Here's how the part is built. I have some questions about the finished solid (model axes, mm). A direction names the side the tool comes from. Coordinates: 2 decimals unless noted, no trailing zeros. Order: outer loops, then holes, each group sorted by start corner. A loop starts at its lowest first (then second) coordinate and runs counter-clockwise, first axis right, second up. Notation, with made-up numbers: (18.25, 53) - (31.25, 53) arc R10 cw to (31.25, 58) - close; hole circle Ø7 at (-26.75, 45.5). An arc over 180 degrees is marked (long way). Answer as CSV lines item,"result". Start each with the question number.
Item 1: I'm going to push flat-ended pins straight in: pin 1 (8 mm diameter, centred on y = 0, z = 15, fed in from +X); pin 2 (5 mm diameter, centred on x = 15, z = 2, fed in from +Y); pin 3 (8 mm diameter, centred on y = -2, z = -6, fed in from +X). Where does each tip first touch, or does it pass through?
Item 2: Imagine slicing it at B-B on y = 42.8. List the corners of the cut face in (x, z) for me, and give its area (3 significant figures).
Item 3: Imagine slicing it at A-A on x = 24. List the corners of the cut face in (y, z) for me, and give its area (3 significant figures).
Item 4: I need wall thicknesses on line 1 (Z direction, x = 2, y = 0); line 2 (Y direction, x = 5, z = 15); line 3 (X direction, y = 1.5, z = 18). Which ranges of each line are inside material? Lowest first, please.
Item 5: Imagine slicing it at C-C on z = -6. List the corners of the cut face in (x, y) for me, and give its area (3 significant figures).
Item 6: We'd pull the mould along Z, two halves only. Please class faces 1 (the face through (24, 0, 32)), 2 (the face through (36, 0, -15)), 3 (the face through (24, 0, -28)): pulls with the +Z half, pulls with the -Z half, needs draft (parallel to the pull), parting line crosses it, or undercut.
Item 7: Imagine slicing it at D-D on x = 10. List the corners of the cut face in (y, z) for me, and give its area (3 significant figures).
Item 8: On a 3-axis mill with a long thin cutter (end or side, diameter ignored), from which of +Z, -Z, +X, -X, +Y, -Y can I reach the whole of each face in a straight line? I mean faces 4 (the face through (12, 0, 0)), 5 (the face through (46.998, 42, 0)), 6 (the face through (48.674, 25.571, 0.14)), 7 (the face through (-1.479, 0.165, 11.254)). Say none if no direction works.
from build123d import *

# Parameters (mm, degrees)
BOSS_EXTRUDE1_DEPTH      = 3.75
SKETCH2_R                = 3.75
BOSS_EXTRUDE2_DEPTH      = 3
M4_CLEARANCE_HOLE1_D     = 4.5
M4_CLEARANCE_HOLE1_DEPTH = 10
M4_CLEARANCE_HOLE1_TIP   = 1.351936393
CUT_EXTRUDE1_DEPTH       = 33
CUT_EXTRUDE1_DEPTH_BACK  = 33
BOSS_EXTRUDE3_DEPTH      = 10
M3_CLEARANCE_HOLE1_D     = 3.4
M3_CLEARANCE_HOLE1_DEPTH = 10
M3_CLEARANCE_HOLE1_TIP   = 1.021463052


with BuildPart() as part:
    # Sketch1 → Boss-Extrude1 (new body, symmetric)
    with BuildSketch(Plane(origin=(0, 0, 0), x_dir=(1, 0, 0), z_dir=(0, 1, 0))):
        with BuildLine():
            Line((0, -11), (12, -11))
            Line((12, -11), (12, 11))
            Line((12, 11), (0, 11))
            Line((0, 11), (0, 19))
            Line((0, 19), (12, 19))
            Line((12, 19), (12, 20))
            ThreePointArc((12, 20), (24, 32), (36, 20))
            Line((36, 20), (36, 10))
            Line((36, 10), (55, 10))
            Line((55, 10), (55, -10))
            Line((55, -10), (36, -10))
            Line((36, -10), (36, -20))
            ThreePointArc((36, -20), (24, -32), (12, -20))
            Line((12, -20), (12, -19))
            Line((12, -19), (0, -19))
            Line((0, -19), (0, -11))
        make_face()
        with BuildLine():
            Line((32, 20), (32, -20))
            ThreePointArc((32, -20), (24, -28), (16, -20))
            Line((16, -20), (16, 20))
            ThreePointArc((16, 20), (24, 28), (32, 20))
        make_face(mode=Mode.SUBTRACT)
    extrude(amount=BOSS_EXTRUDE1_DEPTH, both=True)

    # Sketch2 → Boss-Extrude2 (add)
    with BuildSketch(Plane.ZY):
        with Locations((-15, 0)):
            Circle(SKETCH2_R)
        with Locations((15, 0)):
            Circle(SKETCH2_R)
    extrude(amount=BOSS_EXTRUDE2_DEPTH)

    # M4 Clearance Hole1
    with Locations(Plane.ZY.offset(3)):
        with Locations((-15, 0), (15, 0)):
            Hole(M4_CLEARANCE_HOLE1_D / 2, depth=M4_CLEARANCE_HOLE1_DEPTH)
            with Locations((0, 0, -(M4_CLEARANCE_HOLE1_DEPTH + M4_CLEARANCE_HOLE1_TIP / 2))):  # 118° drill point
                Cone(0, M4_CLEARANCE_HOLE1_D / 2, M4_CLEARANCE_HOLE1_TIP, mode=Mode.SUBTRACT)

    # Sketch6 → Cut-Extrude1 (cut, two sides)
    with BuildSketch(Plane.XY) as cut_extrude1_sk:
        with BuildLine():
            Line((53.548387097, -7.31769585), (58.512723929, -6.476790348))
            Line((58.512723929, -6.476790348), (58.512723929, 16.833295116))
            Line((58.512723929, 16.833295116), (46.662820439, 16.833295116))
            ThreePointArc((46.662820439, 16.833295116), (46.996356715, 3.87133796), (53.548387097, -7.31769585))
        make_face()
    extrude(amount=CUT_EXTRUDE1_DEPTH, mode=Mode.SUBTRACT)
    extrude(cut_extrude1_sk.sketch, amount=-CUT_EXTRUDE1_DEPTH_BACK, mode=Mode.SUBTRACT)

    # Sketch7 → Boss-Extrude3 (add, symmetric)
    with BuildSketch(Plane.XY):
        with BuildLine():
            Line((46.662820439, 16.833295116), (50.743158051, 34.556424956))
            ThreePointArc((50.743158051, 34.556424956), (50.934151856, 35.670993937), (50.998088989, 36.8))
            Line((50.998088989, 36.8), (50.998088989, 53))
            Line((50.998088989, 53), (50.075012066, 52.615384615))
            ThreePointArc((50.075012066, 52.615384615), (47.837837517, 50.773500981), (46.998088989, 48))
            Line((46.998088989, 48), (46.998088989, 36.8))
            ThreePointArc((46.998088989, 36.8), (46.959726709, 36.122596362), (46.845130426, 35.453854973))
            Line((46.845130426, 35.453854973), (42.764792814, 17.730725133))
            ThreePointArc((42.764792814, 17.730725133), (42.138360124, 13.877927021), (42.017467452, 9.976407294))
            ThreePointArc((42.017467452, 9.976407294), (40.329493687, 5.586764491), (36, 3.75))
            Line((36, 3.75), (47.031269556, 3.75))
            ThreePointArc((47.031269556, 3.75), (46.010304001, 10.268083427), (46.662820439, 16.833295116))
        make_face()
    extrude(amount=BOSS_EXTRUDE3_DEPTH, both=True)

    # M3 Clearance Hole1
    with Locations(Plane.ZY.offset(-46.998088989)):
        with Locations((-6, 42.8), (6, 42.8)):
            Hole(M3_CLEARANCE_HOLE1_D / 2, depth=M3_CLEARANCE_HOLE1_DEPTH)
            with Locations((0, 0, -(M3_CLEARANCE_HOLE1_DEPTH + M3_CLEARANCE_HOLE1_TIP / 2))):  # 118° drill point
                Cone(0, M3_CLEARANCE_HOLE1_D / 2, M3_CLEARANCE_HOLE1_TIP, mode=Mode.SUBTRACT)


solid = part.part
Responses:
1,pin 1,"stops at x = 36"
1,pin 2,"stops at y = 3.75"
1,pin 3,"stops at x = 50.59"
2,outline,"(47, -10) - (51, -10) - (51, -7.7) - (47, -7.7) - close; (47, -4.3) - (51, -4.3) - (51, 4.3) - (47, 4.3) - close; (47, 7.7) - (51, 7.7) - (51, 10) - (47, 10) - close"
2,area,"52.8 mm^2"
3,outline,"(-3.75, -32) - (3.75, -32) - (3.75, -28) - (-3.75, -28) - close; (-3.75, 28) - (3.75, 28) - (3.75, 32) - (-3.75, 32) - close"
3,area,"60.0 mm^2"
4,line 1,"z = -19 to -17.25, -12.75 to -11, 11 to 12.75, 17.25 to 19"
4,line 2,"y = -3.75 to -2.25, 2.25 to 3.75"
4,line 3,"x = -3 to 16, 32 to 36"
5,outline,"(12, -3.75) - (16, -3.75) - (16, 3.75) - (12, 3.75) - close; (32, -3.75) - (50.59, -3.75) arc R26 cw to (46.66, 16.83) - (50.74, 34.56) arc R10 ccw to (51, 36.8) - (51, 41.1) - (47, 41.1) - (47, 36.8) arc R6 cw to (46.85, 35.45) - (42.76, 17.73) arc R30 ccw to (42.02, 9.98) arc R6.02 cw to (36, 3.75) - (32, 3.75) - close; (47, 44.5) - (51, 44.5) - (51, 53) - (50.08, 52.62) arc R5 ccw to (47, 48) - close"
5,area,"345 mm^2"
6,face 1,"pulls with the +Z half"
6,face 2,"needs draft"
6,face 3,"undercut"
7,outline,"(-3.75, -19) - (3.75, -19) - (3.75, -11) - (-3.75, -11) - close; (-3.75, 11) - (3.75, 11) - (3.75, 19) - (-3.75, 19) - close"
7,area,"120 mm^2"
8,face 4,"-X, +Y, -Y"
8,face 5,"+Z, -Z, -X, +Y"
8,face 6,"+Z, -Z, +X"
8,face 7,"-X"
